The listing builds one solid part. Answer for the finished solid, in the listing's coordinates (mm). A direction names the side the tool comes from. Round coordinates to 2 decimals unless told otherwise and drop trailing zeros. Loops run counter-clockwise (first coordinate to the right, second up) from the corner with the lowest first, then second, coordinate; pieces in that order, holes last. Notation, with made-up numbers: (-31.75, -12) -> (-17.75, -12) arc R20 ccw to (-17.75, -3) -> close; hole circle Ø11 at (32.25, 38). An arc over 180 degrees is marked (long way). Use a Markdown table: item, result. Add a question column.
Q1. Given pin 1 Ø6 at (y, z) = (0, 1.5) entering from +X; pin 2 Ø1 at (x, z) = (-3, 4) entering from +Y; pin 3 Ø1 at (x, y) = (4.5, 4) entering from -Z, each flat-ended and moving along its own axis, determine where each tip first touches the part or whether it passes through.
Q2. Which of the six approach directions +Z, -Z, +X, -X, +Y, -Y give full straight-line access (tool end or side, diameter ignored) to faces 4 (the flat face through (-4, -2, 10)), 5 (the flat face through (2, -5, 7))?
Q3. Section A-A on x = 0 is taken. Give the vertices of the cut face in (y, z).
Q4. For a pull along Y with two mould halves and no side action, classify faces 1 (the cylindrical face through (-5.158, -3.955, 7.986)), 2 (the flat face through (1, -3, 0)), 3 (the cylindrical face through (-3, 0, 4)) as released by +Y, released by -Y, zero draft, split by the parting line, or undercut.
Q5. Section D-D on z = 2 is taken. Give the vertices of the cut face in (x, y).
Q6. Section C-C on z = 7.5 is taken. Give the vertices of the cut face in (x, y), then the cut area to 3 significant figures.
Q7. Consider line 1 (Y direction, x = 0, z = 6); line 2 (Y direction, x = -0.25, z = 9); line 3 (X direction, y = 2.5, z = 1). Determine where each line is inside the solid, lowest interval first.
from build123d import *

# Parameters (mm, degrees)
SKETCH1_R           = 5
SKETCH1_R_2         = 3
BOSS_EXTRUDE1_DEPTH = 7
SKETCH2_R           = 6.5
SKETCH2_R_2         = 3
BOSS_EXTRUDE2_DEPTH = 3
FILLET1_R           = 1
FILLET2_R           = 0.5


with BuildPart() as part:
    # Sketch1 → Boss-Extrude1 (new body)
    with BuildSketch(Plane.XY):
        Circle(SKETCH1_R)
        Circle(SKETCH1_R_2, mode=Mode.SUBTRACT)
    extrude(amount=BOSS_EXTRUDE1_DEPTH)

    # Sketch2 → Boss-Extrude2 (add)
    with BuildSketch(Plane.XY.offset(7)):
        Circle(SKETCH2_R)
        Circle(SKETCH2_R_2, mode=Mode.SUBTRACT)
    extrude(amount=BOSS_EXTRUDE2_DEPTH)

    # Fillet1
    fillet1_edges = [part.edges().sort_by_distance(p)[0] for p in [
        (-6.5, 0, 10),
        (-3, 0, 10),
    ]]
    fillet(fillet1_edges, radius=FILLET1_R)

    # Fillet2
    fillet2_edges = [part.edges().sort_by_distance(p)[0] for p in [
        (-5, 0, 0),
    ]]
    fillet(fillet2_edges, radius=FILLET2_R)


solid = part.part
Checked values:
| question | item | result |
|---|---|---|
| 1 | pin 1 | stops at x = 5 |
| 1 | pin 2 | stops at y = 4.33 |
| 1 | pin 3 | stops at z = 7 |
| 2 | face 4 | +Z, +X, -X, +Y, -Y |
| 2 | face 5 | -Z |
| 3 | outline | (-6.5, 7) -> (-5, 7) -> (-5, 0.5) arc R0.5 ccw to (-4.5, 0) -> (-3, 0) -> (-3, 9) arc R1 ccw to (-4, 10) -> (-5.5, 10) arc R1 ccw to (-6.5, 9) -> close; (3, 0) -> (4.5, 0) arc R0.5 ccw to (5, 0.5) -> (5, 7) -> (6.5, 7) -> (6.5, 9) arc R1 ccw to (5.5, 10) -> (4, 10) arc R1 ccw to (3, 9) -> close |
| 4 | face 1 | split by the parting line |
| 4 | face 2 | zero draft |
| 4 | face 3 | undercut |
| 5 | outline | circle Ø10 at (0, 0); hole circle Ø6 at (0, 0) |
| 6 | outline | circle Ø13 at (0, 0); hole circle Ø6 at (0, 0) |
| 6 | area | 104 mm2 |
| 7 | line 1 | y = -5 to -3, 3 to 5 |
| 7 | line 2 | y = -6.5 to -2.99, 2.99 to 6.5 |
| 7 | line 3 | x = -4.33 to -1.66, 1.66 to 4.33 |
